Input: part model. Units: mm. Frame: model coordinates. Round coordinates to 2 decimals unless told otherwise and drop trailing zeros. Order: outer loops, then holes, each group sorted by start corner. A loop starts at its lowest first (then second) coordinate and runs counter-clockwise, first axis right, second up. Notation, with made-up numbers: (50, -12) -> (108, -12) arc R10 cw to (108, 6) -> close; hole circle Ø5 at (48, -10). An arc over 180 degrees is marked (long way). Answer as CSV lines item,"result". Start each with the question number.
1) Section query C-C, the plane x = -6.35. Output: boundary loops of the cut face in (y, z) (3 decimals).
2) First-contact query: P1, Ø2.5, axis at x = -38.54, z = 18.03, coming from the +Y side. Flat tip, straight axial feed; report the tip coordinate or a pass-through.
3) Line query: L1, parallel to Z at x = -82.55, y = 1.8; L2, parallel to X at y = 1.65, z = -10; L3, parallel to X at y = 2.15, z = -24.5. Output: solid intervals per line, ascending.
4) Section query B-B, the plane x = -82.55. Output: boundary loops of the cut face in (y, z) (3 decimals), and give its area (3 significant figures).
5) Section query A-A, the plane z = 22.86. Output: boundary loops of the cut face in (x, y) (1 decimal), and give its area (3 significant figures).
```python
from build123d import *

# Parameters (mm, degrees)
BASE_SKETCH_W                              = 174.625
BASE_SKETCH_H                              = 76.2
BASE_PLATE_DEPTH                           = 3.175
F_4_40_GUIDE_RAIL_HOLES_REACH              = 97.316
F_4_40_HOLE_PATTERN_SKETCH_GUIDE_RAIL_R    = 1.7145
F_4_40_ARDUINO_HOLES_REACH                 = 97.316
F_4_40_HOLE_PATTERN_SKETCH_ARDUINO_HOLES_R = 1.7145
F_4_40_IMU_MOUNT_HOLES_REACH               = 97.316
F_4_40_HOLE_PATTERN_SKETCH_IMU_MOUNT_R     = 1.7145


with BuildPart() as part:
    # Base Sketch → Base Plate (new body)
    with BuildSketch(Plane(origin=(0, 0, 0), x_dir=(1, 0, 0), z_dir=(0, 1, 0))):
        Rectangle(BASE_SKETCH_W, BASE_SKETCH_H)
    extrude(amount=BASE_PLATE_DEPTH)

    # 4-40 Hole Pattern Sketch (Guide Rail) → 4-40 Guide Rail Holes (cut, up to next)
    with BuildSketch(Plane(origin=(0, 3.175, 0), x_dir=(1, 0, 0), z_dir=(0, 1, 0)), mode=Mode.PRIVATE) as f_4_40_guide_rail_holes_sk1:
        with Locations(Location((-82.55, 33.3375, 0), (0, 0, 270))):
            Circle(F_4_40_HOLE_PATTERN_SKETCH_GUIDE_RAIL_R)
    f_4_40_guide_rail_holes_tool1 = extrude(f_4_40_guide_rail_holes_sk1.sketch, amount=-F_4_40_GUIDE_RAIL_HOLES_REACH, mode=Mode.PRIVATE) & part.part
    # 4-40 Hole Pattern Sketch (Guide Rail) → 4-40 Guide Rail Holes (cut, up to next)
    with BuildSketch(Plane(origin=(0, 3.175, 0), x_dir=(1, 0, 0), z_dir=(0, 1, 0)), mode=Mode.PRIVATE) as f_4_40_guide_rail_holes_sk2:
        with Locations(Location((-82.55, -33.3375, 0), (0, 0, 270))):
            Circle(F_4_40_HOLE_PATTERN_SKETCH_GUIDE_RAIL_R)
    f_4_40_guide_rail_holes_tool2 = extrude(f_4_40_guide_rail_holes_sk2.sketch, amount=-F_4_40_GUIDE_RAIL_HOLES_REACH, mode=Mode.PRIVATE) & part.part
    # 4-40 Hole Pattern Sketch (Guide Rail) → 4-40 Guide Rail Holes (cut, up to next)
    with BuildSketch(Plane(origin=(0, 3.175, 0), x_dir=(1, 0, 0), z_dir=(0, 1, 0)), mode=Mode.PRIVATE) as f_4_40_guide_rail_holes_sk3:
        with Locations(Location((-6.35, 33.3375, 0), (0, 0, 270))):
            Circle(F_4_40_HOLE_PATTERN_SKETCH_GUIDE_RAIL_R)
    f_4_40_guide_rail_holes_tool3 = extrude(f_4_40_guide_rail_holes_sk3.sketch, amount=-F_4_40_GUIDE_RAIL_HOLES_REACH, mode=Mode.PRIVATE) & part.part
    add(f_4_40_guide_rail_holes_tool1.solids().sort_by_distance((-82.55, 3.175, -33.3375))[0], mode=Mode.SUBTRACT)
    add(f_4_40_guide_rail_holes_tool2.solids().sort_by_distance((-82.55, 3.175, 33.3375))[0], mode=Mode.SUBTRACT)
    add(f_4_40_guide_rail_holes_tool3.solids().sort_by_distance((-6.35, 3.175, -33.3375))[0], mode=Mode.SUBTRACT)

    # 4-40 Hole Pattern Sketch (Arduino Holes) → 4-40 Arduino Holes (cut, up to next)
    with BuildSketch(Plane(origin=(0, 3.175, 0), x_dir=(1, 0, 0), z_dir=(0, 1, 0)), mode=Mode.PRIVATE) as f_4_40_arduino_holes_sk1:
        with Locations(Location((-38.5445, -18.034, 0), (0, 0, 270))):
            Circle(F_4_40_HOLE_PATTERN_SKETCH_ARDUINO_HOLES_R)
    f_4_40_arduino_holes_tool1 = extrude(f_4_40_arduino_holes_sk1.sketch, amount=-F_4_40_ARDUINO_HOLES_REACH, mode=Mode.PRIVATE) & part.part
    # 4-40 Hole Pattern Sketch (Arduino Holes) → 4-40 Arduino Holes (cut, up to next)
    with BuildSketch(Plane(origin=(0, 3.175, 0), x_dir=(1, 0, 0), z_dir=(0, 1, 0)), mode=Mode.PRIVATE) as f_4_40_arduino_holes_sk2:
        with Locations(Location((-38.5445, 9.906, 0), (0, 0, 270))):
            Circle(F_4_40_HOLE_PATTERN_SKETCH_ARDUINO_HOLES_R)
    f_4_40_arduino_holes_tool2 = extrude(f_4_40_arduino_holes_sk2.sketch, amount=-F_4_40_ARDUINO_HOLES_REACH, mode=Mode.PRIVATE) & part.part
    # 4-40 Hole Pattern Sketch (Arduino Holes) → 4-40 Arduino Holes (cut, up to next)
    with BuildSketch(Plane(origin=(0, 3.175, 0), x_dir=(1, 0, 0), z_dir=(0, 1, 0)), mode=Mode.PRIVATE) as f_4_40_arduino_holes_sk3:
        with Locations(Location((-69.5325, -22.86, 0), (0, 0, 270))):
            Circle(F_4_40_HOLE_PATTERN_SKETCH_ARDUINO_HOLES_R)
    f_4_40_arduino_holes_tool3 = extrude(f_4_40_arduino_holes_sk3.sketch, amount=-F_4_40_ARDUINO_HOLES_REACH, mode=Mode.PRIVATE) & part.part
    # 4-40 Hole Pattern Sketch (Arduino Holes) → 4-40 Arduino Holes (cut, up to next)
    with BuildSketch(Plane(origin=(0, 3.175, 0), x_dir=(1, 0, 0), z_dir=(0, 1, 0)), mode=Mode.PRIVATE) as f_4_40_arduino_holes_sk4:
        with Locations(Location((-62.0395, 25.4762, 0), (0, 0, 270))):
            Circle(F_4_40_HOLE_PATTERN_SKETCH_ARDUINO_HOLES_R)
    f_4_40_arduino_holes_tool4 = extrude(f_4_40_arduino_holes_sk4.sketch, amount=-F_4_40_ARDUINO_HOLES_REACH, mode=Mode.PRIVATE) & part.part
    add(f_4_40_arduino_holes_tool1.solids().sort_by_distance((-38.5445, 3.175, 18.034))[0], mode=Mode.SUBTRACT)
    add(f_4_40_arduino_holes_tool2.solids().sort_by_distance((-38.5445, 3.175, -9.906))[0], mode=Mode.SUBTRACT)
    add(f_4_40_arduino_holes_tool3.solids().sort_by_distance((-69.5325, 3.175, 22.86))[0], mode=Mode.SUBTRACT)
    add(f_4_40_arduino_holes_tool4.solids().sort_by_distance((-62.0395, 3.175, -25.4762))[0], mode=Mode.SUBTRACT)

    # 4-40 Hole Pattern Sketch (IMU Mount) → 4-40 IMU Mount Holes (cut, up to next)
    with BuildSketch(Plane(origin=(0, 3.175, 0), x_dir=(1, 0, 0), z_dir=(0, 1, 0)), mode=Mode.PRIVATE) as f_4_40_imu_mount_holes_sk1:
        with Locations(Location((82.2325, -33.02, 0), (0, 0, 270))):
            Circle(F_4_40_HOLE_PATTERN_SKETCH_IMU_MOUNT_R)
    f_4_40_imu_mount_holes_tool1 = extrude(f_4_40_imu_mount_holes_sk1.sketch, amount=-F_4_40_IMU_MOUNT_HOLES_REACH, mode=Mode.PRIVATE) & part.part
    # 4-40 Hole Pattern Sketch (IMU Mount) → 4-40 IMU Mount Holes (cut, up to next)
    with BuildSketch(Plane(origin=(0, 3.175, 0), x_dir=(1, 0, 0), z_dir=(0, 1, 0)), mode=Mode.PRIVATE) as f_4_40_imu_mount_holes_sk2:
        with Locations(Location((54.2925, -33.02, 0), (0, 0, 270))):
            Circle(F_4_40_HOLE_PATTERN_SKETCH_IMU_MOUNT_R)
    f_4_40_imu_mount_holes_tool2 = extrude(f_4_40_imu_mount_holes_sk2.sketch, amount=-F_4_40_IMU_MOUNT_HOLES_REACH, mode=Mode.PRIVATE) & part.part
    # 4-40 Hole Pattern Sketch (IMU Mount) → 4-40 IMU Mount Holes (cut, up to next)
    with BuildSketch(Plane(origin=(0, 3.175, 0), x_dir=(1, 0, 0), z_dir=(0, 1, 0)), mode=Mode.PRIVATE) as f_4_40_imu_mount_holes_sk3:
        with Locations(Location((39.0525, -8.636, 0), (0, 0, 270))):
            Circle(F_4_40_HOLE_PATTERN_SKETCH_IMU_MOUNT_R)
    f_4_40_imu_mount_holes_tool3 = extrude(f_4_40_imu_mount_holes_sk3.sketch, amount=-F_4_40_IMU_MOUNT_HOLES_REACH, mode=Mode.PRIVATE) & part.part
    add(f_4_40_imu_mount_holes_tool1.solids().sort_by_distance((82.2325, 3.175, 33.02))[0], mode=Mode.SUBTRACT)
    add(f_4_40_imu_mount_holes_tool2.solids().sort_by_distance((54.2925, 3.175, 33.02))[0], mode=Mode.SUBTRACT)
    add(f_4_40_imu_mount_holes_tool3.solids().sort_by_distance((39.0525, 3.175, 8.636))[0], mode=Mode.SUBTRACT)


solid = part.part
```
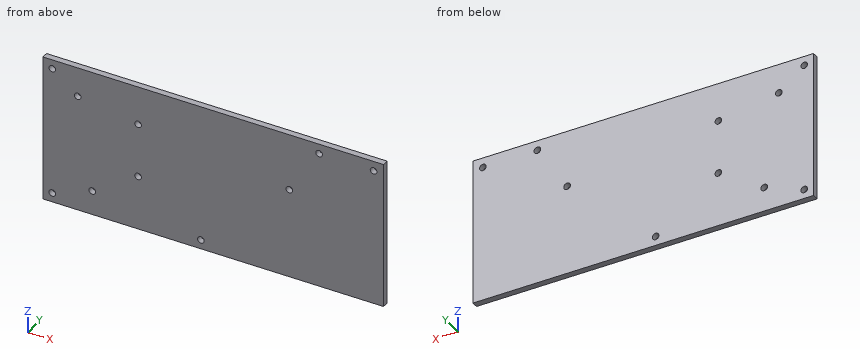
Findings:
1,outline,"(0, -38.1) -> (3.175, -38.1) -> (3.175, -35.052) -> (0, -35.052) -> close; (0, -31.623) -> (3.175, -31.623) -> (3.175, 38.1) -> (0, 38.1) -> close"
2,P1,"passes through"
3,L1,"z = -38.1 to -35.05, -31.62 to 31.62, 35.05 to 38.1"
3,L2,"x = -87.31 to -40.26, -36.83 to 87.31"
3,L3,"x = -87.31 to -63.45, -60.63 to 87.31"
4,outline,"(0, -38.1) -> (3.175, -38.1) -> (3.175, -35.052) -> (0, -35.052) -> close; (0, -31.623) -> (3.175, -31.623) -> (3.175, 31.623) -> (0, 31.623) -> close; (0, 35.052) -> (3.175, 35.052) -> (3.175, 38.1) -> (0, 38.1) -> close"
4,area,"220 mm^2"
5,outline,"(-87.3, 0) -> (-71.2, 0) -> (-71.2, 3.2) -> (-87.3, 3.2) -> close; (-67.8, 0) -> (87.3, 0) -> (87.3, 3.2) -> (-67.8, 3.2) -> close"
5,area,"544 mm^2"
